Build history of the part. All positions in model axes, mm. A direction names the side the tool comes from. Round coordinates to 2 decimals unless told otherwise and drop trailing zeros. Write each loop counter-clockwise with the first axis right and the second up, starting at its lowest first coordinate (ties: lowest second). Pieces come first, ordered by that corner, then holes. Notation, with made-up numbers: M -28.5,59.25 L -15.5,59.25 A30 cw -15.5,91.25 Z; hole C 56.5,-26 d7. An arc over 180 degrees is marked long. Write item = value, one per line.
from build123d import *

# Parameters (mm, degrees)
SKETCH_W             = 18
SKETCH_H             = 18
PAD_DEPTH            = 8
POCKET_DEPTH         = 18.001
POCKET001_DEPTH      = 9.001
POCKET001_DEPTH_BACK = 9.001
FILLET_R             = 2
THICKNESS_T          = -1
POCKET002_DEPTH      = 1


with BuildPart() as part:
    # Sketch → Pad (new body)
    with BuildSketch(Plane.XY):
        Rectangle(SKETCH_W, SKETCH_H)
    extrude(amount=PAD_DEPTH)

    # Sketch001 (on Face1 of Pad) → Pocket (cut, through all)
    with BuildSketch(Plane.XZ.offset(9)):
        Polygon((-9, 8), (-9, 0), (-7, 8), align=None)
        Polygon((9, 8), (9, 0), (7, 8), align=None)
    extrude(amount=-POCKET_DEPTH, mode=Mode.SUBTRACT)

    # Sketch002 → Pocket001 (cut, two sides)
    with BuildSketch(Plane.YZ) as pocket001_sk:
        Polygon((-9, 8), (-7, 8), (-9, 0), align=None)
        Polygon((9, 8), (7, 8), (9, 0), align=None)
    extrude(amount=-POCKET001_DEPTH, mode=Mode.SUBTRACT)
    extrude(pocket001_sk.sketch, amount=POCKET001_DEPTH_BACK, mode=Mode.SUBTRACT)

    # Fillet
    fillet_edges = [part.edges().sort_by_distance(p)[0] for p in [
        (-8, 8, 4),
        (-8, -8, 4),
        (8, -8, 4),
        (8, 8, 4),
    ]]
    fillet(fillet_edges, radius=FILLET_R)

    # Thickness
    thickness_openings = [part.faces().sort_by_distance(p)[0] for p in [
        (0, 0, 0),
    ]]
    offset(amount=THICKNESS_T, openings=thickness_openings, kind=Kind.INTERSECTION)

    # Sketch003 (on Face9 of Thickness) → Pocket002 (cut)
    with BuildSketch(Plane.XY.offset(8)):
        with BuildLine():
            ThreePointArc((-4.383089, -3.322429), (-3.889087, -3.889087), (-3.322429, -4.383089))
            Line((-3.322429, -4.383089), (4.383089, 3.322429))
            ThreePointArc((4.383089, 3.322429), (3.889087, 3.889087), (3.322429, 4.383089))
            Line((3.322429, 4.383089), (-4.383089, -3.322429))
        make_face()
        with BuildLine():
            ThreePointArc((-1.305937, -3.780811), (2.828427, -2.828427), (3.780811, 1.305937))
            Line((4.924407, 2.449533), (3.780811, 1.305937))
            ThreePointArc((-2.449533, -4.924407), (3.889087, -3.889087), (4.924407, 2.449533))
            Line((-1.305937, -3.780811), (-2.449533, -4.924407))
        make_face()
        with BuildLine():
            Line((-4.924407, -2.449533), (-3.780811, -1.305937))
            ThreePointArc((1.305937, 3.780811), (-2.828427, 2.828427), (-3.780811, -1.305937))
            Line((1.305937, 3.780811), (2.449533, 4.924407))
            ThreePointArc((2.449533, 4.924407), (-3.889087, 3.889087), (-4.924407, -2.449533))
        make_face()
    extrude(amount=-POCKET002_DEPTH, mode=Mode.SUBTRACT)


solid = part.part
1. Band-saw the part on B-B (z = 7.25). Count the separate pieces of the cut face and the enclosed holes in it, plus the area to 3 significant figures.
Responses:
separate_pieces = 1
enclosed_holes = 3
area = 153 mm²
2. Flat gauge pins, fed straight in: pin 1 (2 mm diameter, centred on y = 6.5, z = 3, fed in from -X); pin 2 (2 mm diameter, centred on x = -2, z = 6, fed in from +Y). Where does each tip first touch, or does it go through?
Responses:
pin_1 = -8.5
pin_2 = 7.75
3. Band-saw the part on A-A (x = 0). List the corners of the cut face in (y, z), plus the area to 3 significant figures.
Responses:
outline = M -9,0 L -7.97,0 L -6.22,7 L -5.5,7 L -5.5,8 L -7,8 Z; M -4,7 L -1.06,7 L -1.06,8 L -4,8 Z; M 1.06,7 L 4,7 L 4,8 L 1.06,8 Z; M 5.5,7 L 6.22,7 L 7.97,0 L 9,0 L 7,8 L 5.5,8 Z
area = 23.6 mm²
4. Mould opens along X. For faces 4 (the face through (-7.424, 7.454, 3.997)), 5 (the face through (7.395, 7.425, 4.112)), 6 (the face through (-2.784, 2.872, 7.507)), 7 (the face through (-0.48, 0.58, 7.51)) say: pulls with the +X half, pulls with the -X half, needs draft (parallel to the pull), parting line crosses it, or undercut.
Responses:
face_4 = pulls with the -X half
face_5 = pulls with the +X half
face_6 = undercut
face_7 = undercut
5. Probe probe 1 along Z at (x, y) = (-5.75, -2); probe 2 along X at (y, z) = (5.75, 4); probe 3 along X at (y, z) = (1, 6.5) (3 decimals). List the from-to ranges inside material, lowest first.
Responses:
probe_1 = 7 to 8
probe_2 = -8 to -6.97, 6.97 to 8
probe_3 = -7.375 to -6.344, 6.344 to 7.375
6. Tool access for faces 1 (the face through (7.425, -7.395, 4.112)), 2 (the face through (-6.81, 6.82, 3.49)), 3 (the face through (-4.361, -1.886, 7.507)): list every direction of +Z, -Z, +X, -X, +Y, -Y with a clear straight run to the whole face (end or side of a thin tool).
Responses:
face_1 = +Z, +X, -Y
face_2 = -Z
face_3 = +Z, -Z
